from build123d import *

# Parameters (mm, degrees)
BOSS_EXTRUDE1_DEPTH = 10
SKETCH2_R           = 1.7
CUT_EXTRUDE1_DEPTH  = 21.081085628
FILLET1_R           = 1


with BuildPart() as part:
    # Sketch1 → Boss-Extrude1 (new body)
    with BuildSketch(Plane.XY):
        with BuildLine():
            Line((-13.5, 0), (-13.5, 1.5))
            Line((-13.5, 1.5), (-7, 1.5))
            Line((-7, 1.5), (-7, 5.5))
            ThreePointArc((-7, 5.5), (0, 12.5), (7, 5.5))
            Line((7, 5.5), (7, 1.5))
            Line((7, 1.5), (13.5, 1.5))
            Line((13.5, 1.5), (13.5, 0))
            Line((13.5, 0), (5.5, 0))
            Line((5.5, 0), (5.5, 5.5))
            ThreePointArc((5.5, 5.5), (0, 11), (-5.5, 5.5))
            Line((-5.5, 5.5), (-5.5, 0))
            Line((-5.5, 0), (-13.5, 0))
        make_face()
    extrude(amount=BOSS_EXTRUDE1_DEPTH)

    # Sketch2 → Cut-Extrude1 (cut, through all)
    with BuildSketch(Plane(origin=(0, 1.5, 0), x_dir=(1, 0, 0), z_dir=(0, 1, 0))):
        with Locations(Location((10.25, -5, 0), (0, 0, 180))):
            Circle(SKETCH2_R)
    cut_extrude1 = extrude(amount=-CUT_EXTRUDE1_DEPTH, mode=Mode.SUBTRACT)

    # Fillet1
    fillet1_edges = [part.edges().sort_by_distance(p)[0] for p in [
        (-7, 1.5, 5),
        (7, 1.5, 5),
    ]]
    fillet(fillet1_edges, radius=FILLET1_R)

    # Mirror1: Cut-Extrude1 across plane
    add(cut_extrude1.mirror(Plane(origin=(0, 0, 0), x_dir=(0, 0, 1), z_dir=(1, 0, 0))), mode=Mode.SUBTRACT)


solid = part.part
Can you work these out from the model? Positions are in its coordinate system, mm. A direction names the side the tool comes from. Round coordinates to 2 decimals unless told otherwise and drop trailing zeros. Loops run counter-clockwise (first coordinate to the right, second up) from the corner with the lowest first, then second, coordinate; pieces in that order, holes last. Notation, with made-up numbers: (18, 63.5) - (35, 63.5) arc R25 cw to (35, 77.5) - close; hole circle Ø7 at (-38, 57.25). An arc over 180 degrees is marked (long way). Use CSV: the item, a comma, the result in double quotes. Start each with the question number.
1) For pin 1 Ø3.5 at (y, z) = (3.5, 6.5) entering from +X; pin 2 Ø4.5 at (x, z) = (10.25, 5) entering from +Y; pin 3 Ø1.5 at (y, z) = (11, 4.5) entering from -X, each with a flat end and sliding along its axis, tell me the tip position at first contact or that it passes through.
2) If we section it at B-B on z = 6: Write out the boundary of the cut face in (x, y).
3) Please list where these lines run through material, in increasing order: probe 1 along Z at (x, y) = (10.25, 0.95); probe 2 along X at (y, z) = (3.25, 1.5); probe 3 along X at (y, z) = (10.5, 5.5). Write a range as [from, to].
4) If we section it at D-D on z = 1: Write out the boundary of the cut face in (x, y), plus the area to 3 significant figures.
5) For faces 5 (the cylindrical face through (9.47, 0.76, 3.49)), 6 (the flat face through (-5.5, 3, 5)), 7 (the flat face through (-7, 4, 5)), 8 (the flat face through (7, 4, 5)), 9 (the flat face through (-13.5, 1, 5)), which set-ups out of +Z, -Z, +X, -X, +Y, -Y let a thin tool reach every point of the face, with its end or its side?
6) We'd pull the mould along Z, two halves only. Please class faces 1 (the flat face through (-6, 5, 0)), 2 (the flat face through (8.7, 0, 3.8)), 3 (the flat face through (-6, 5, 10)), 4 (the cylindrical face through (-9.47, 0.76, 3.49)): released by +Z, released by -Z, zero draft, split by the parting line, or undercut.
7) If we section it at A-A on x = 10.25: Write out the boundary of the cut face in (y, z), plus the area to 3 significant figures.
8) If we section it at C-C on y = 2: Write out the boundary of the cut face in (x, z), plus the area to 3 significant figures.
Geometry results:
1,pin 1,"stops at x = 7.34"
1,pin 2,"stops at y = 1.5"
1,pin 3,"stops at x = -5.14"
2,outline,"(-13.5, 0) - (-11.62, 0) - (-11.62, 1.5) - (-13.5, 1.5) - close; (-8.88, 0) - (-5.5, 0) - (-5.5, 5.5) arc R5.5 cw to (5.5, 5.5) - (5.5, 0) - (8.88, 0) - (8.88, 1.5) - (8, 1.5) arc R1 cw to (7, 2.5) - (7, 5.5) arc R7 ccw to (-7, 5.5) - (-7, 2.5) arc R1 cw to (-8, 1.5) - (-8.88, 1.5) - close; (11.62, 0) - (13.5, 0) - (13.5, 1.5) - (11.62, 1.5) - close"
3,probe 1,"z = [0, 3.3], [6.7, 10]"
3,probe 2,"x = [-7, -5.5], [5.5, 7]"
3,probe 3,"x = [-4.9, -2.29], [2.29, 4.9]"
4,outline,"(-13.5, 0) - (-5.5, 0) - (-5.5, 5.5) arc R5.5 cw to (5.5, 5.5) - (5.5, 0) - (13.5, 0) - (13.5, 1.5) - (8, 1.5) arc R1 cw to (7, 2.5) - (7, 5.5) arc R7 ccw to (-7, 5.5) - (-7, 2.5) arc R1 cw to (-8, 1.5) - (-13.5, 1.5) - close"
4,area,"65.9 mm2"
5,face 5,"+Y, -Y"
5,face 6,"+Z, -Z, -Y"
5,face 7,"+Z, -Z, -X, +Y"
5,face 8,"+Z, -Z, +X, +Y"
5,face 9,"+Z, -Z, -X, +Y, -Y"
6,face 1,"released by -Z"
6,face 2,"zero draft"
6,face 3,"released by +Z"
6,face 4,"undercut"
7,outline,"(0, 0) - (1.5, 0) - (1.5, 3.3) - (0, 3.3) - close; (0, 6.7) - (1.5, 6.7) - (1.5, 10) - (0, 10) - close"
7,area,"9.90 mm2"
8,outline,"(-7.13, 0) - (-5.5, 0) - (-5.5, 10) - (-7.13, 10) - close; (5.5, 0) - (7.13, 0) - (7.13, 10) - (5.5, 10) - close"
8,area,"32.7 mm2"
